The figure shows three views and two pictorial views of one solid part (mm, origin at its lowest corner). Answer the questions. A direction names the side the tool comes from. Give positions to 0.01 mm unless a question says otherwise; leave off trailing zeros. Order: outer loops, then holes, each group sorted by start corner. A loop starts at its lowest first (then second) coordinate and runs counter-clockwise, first axis right, second up. Notation, with made-up numbers: (-10, -24) - (8, -24) arc R20 ccw to (8, -19) - close; hole circle Ø7 at (47.5, 88.25). An arc over 180 degrees is marked (long way). Answer as a JSON object with one key per item and string values. Group by question number.
Q1. A cutting plane is placed at C-C, the plane x = 52.5. Give the vertices of the cut face in (y, z).
Q2. A cutting plane is placed at A-A, the plane x = 71. Give the vertices of the cut face in (y, z).
Q3. Consider line 1 (X direction, y = 11, z = 91.5); line 2 (Z direction, x = 45.5, y = 33); line 3 (Z direction, x = 63, y = 28.5). Determine where each line is inside the solid, lowest interval first.
Q4. A cutting plane is placed at B-B, the plane y = 56.5. Give the vertices of the cut face in (x, z), and give its area (3 significant figures).
Q5. Given pin 1 (6 mm diameter, centred on x = 44, z = 118, fed in from +Y); pin 2 (5 mm diameter, centred on x = 62.5, y = 33, fed in from -Z); pin 3 (10 mm diameter, centred on y = 20.5, z = 145, fed in from +X); pin 4 (2 mm diameter, centred on y = 10.5, z = 165, fed in from -X), each flat-ended and moving along its own axis, determine where each tip first touches the part or whether it passes through.
Q6. A cutting plane is placed at D-D, the plane z = 52. Give the vertices of the cut face in (x, y).
Q7. The mould has two halves that part along Z. Classify the marked faces 1, 2 and 3: released by +Z, released by -Z, zero draft, split by the parting line, or undercut.
Q8. For the marked faces 4 and 5, determine the directions among +Z, -Z, +X, -X, +Y, -Y from which every point of the face is accessible in a straight line to the end or side of a thin tool.
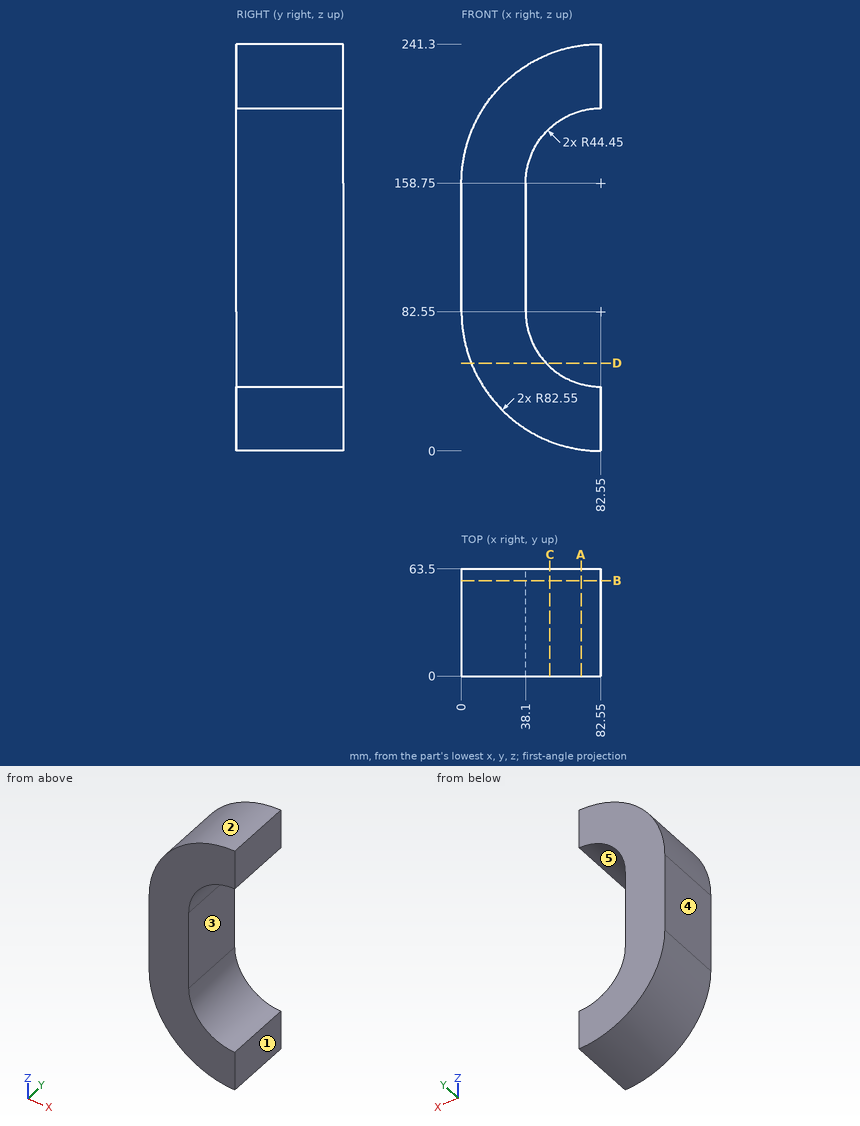
Reply:
{
 "1": {"outline": "(0, 5.66) - (63.5, 5.66) - (63.5, 49.8) - (0, 49.8) - close; (0, 191.5) - (63.5, 191.5) - (63.5, 235.64) - (0, 235.64) - close"},
 "2": {"outline": "(0, 0.81) - (63.5, 0.81) - (63.5, 39.63) - (0, 39.63) - close; (0, 201.67) - (63.5, 201.67) - (63.5, 240.49) - (0, 240.49) - close"},
 "3": {"line 1": "x = 0 to 38.1", "line 2": "z = 8.78 to 57.99, 183.31 to 232.52", "line 3": "z = 2.35 to 42.63, 198.67 to 238.95"},
 "4": {"outline": "(0, 82.55) arc R82.55 ccw to (82.55, 0) - (82.55, 38.1) arc R44.45 cw to (38.1, 82.55) - (38.1, 158.75) arc R44.45 cw to (82.55, 203.2) - (82.55, 241.3) arc R82.55 ccw to (0, 158.75) - close", "area": "10,500 mm^2"},
 "5": {"pin 1": "passes through", "pin 2": "stops at z = 1.89", "pin 3": "stops at x = 38.1", "pin 4": "stops at x = 0.17"},
 "6": {"outline": "(5.86, 0) - (50.26, 0) - (50.26, 63.5) - (5.86, 63.5) - close"},
 "7": {"face 1": "zero draft", "face 2": "released by +Z", "face 3": "undercut"},
 "8": {"face 4": "+Z, -Z, -X, +Y, -Y", "face 5": "+X, +Y, -Y"}
}
